Read the model definition and answer for the solid it produces. Units are mm, in the model's axes. Coordinates: 2 decimals unless noted, no trailing zeros. Write each loop counter-clockwise with the first axis right and the second up, starting at its lowest first coordinate (ties: lowest second). Pieces come first, ordered by that corner, then holes.
(1) Straight lines are drawn through the part: line 1 along X through (y, z) = (3.4, 0); line 2 along X through (y, z) = (-3.5, 0.75); line 3 along Z through (x, y) = (-35, 1). For each, find the intervals that lie inside material, in ascending order.
(2) The part is cut by section C-C, the plane y = 1.25. Determine the outline of the cut face in (x, z) (1 decimal).
(3) The part is cut by section A-A, the plane z = 0. Determine the outline of the cut face in (x, y) (1 decimal), and give its area (3 significant figures).
(4) The part is cut by section B-B, the plane x = -8. Determine the outline of the cut face in (y, z) (3 decimals).
(5) Given pin 1 (3 mm diameter, centred on x = -19, z = -3, fed in from +Y); pin 2 (3.5 mm diameter, centred on x = 35.306, z = 0, fed in from +Y) (3 decimals); pin 3 (2 mm diameter, centred on x = 28.5, z = -3, fed in from -Y); pin 4 (1.5 mm diameter, centred on x = -2.5, y = 1, fed in from +Z), each flat-ended and moving along its own axis, determine where each tip first touches the part or whether it passes through.
```python
from build123d import *

# Parameters (mm, degrees)
SKETCH1_R               = 4.445
BOSS_EXTRUDE1_DEPTH     = 38.481
SKETCH2_R               = 1.5875
CUT_EXTRUDE1_DEPTH      = 5.445
CUT_EXTRUDE1_DEPTH_BACK = 5.445


with BuildPart() as part:
    # Sketch1 → Boss-Extrude1 (new body, symmetric)
    with BuildSketch(Plane(origin=(0, 0, 0), x_dir=(0, 0, -1), z_dir=(1, 0, 0))):
        Circle(SKETCH1_R)
    extrude(amount=BOSS_EXTRUDE1_DEPTH, both=True)

    # Sketch2 → Cut-Extrude1 (cut, two sides)
    with BuildSketch(Plane(origin=(0, 0, 0), x_dir=(1, 0, 0), z_dir=(0, 1, 0))) as cut_extrude1_sk:
        with Locations((-35.306, 0)):
            Circle(SKETCH2_R)
        with Locations((35.306, 0)):
            Circle(SKETCH2_R)
    extrude(amount=CUT_EXTRUDE1_DEPTH, mode=Mode.SUBTRACT)
    extrude(cut_extrude1_sk.sketch, amount=-CUT_EXTRUDE1_DEPTH_BACK, mode=Mode.SUBTRACT)


solid = part.part
```
Computed:
1. line 1: x = -38.48 to -36.89, -33.72 to 33.72, 36.89 to 38.48
1. line 2: x = -38.48 to -36.71, -33.91 to 33.91, 36.71 to 38.48
1. line 3: z = -4.33 to -1.56, 1.56 to 4.33
2. outline: (-38.5, -4.3) - (38.5, -4.3) - (38.5, 4.3) - (-38.5, 4.3) - close; hole circle Ø3.2 at (-35.3, 0); hole circle Ø3.2 at (35.3, 0)
3. outline: (-38.5, -4.4) - (-36.9, -4.4) - (-36.9, 4.4) - (-38.5, 4.4) - close; (-33.7, -4.4) - (33.7, -4.4) - (33.7, 4.4) - (-33.7, 4.4) - close; (36.9, -4.4) - (38.5, -4.4) - (38.5, 4.4) - (36.9, 4.4) - close
3. area: 628 mm2
4. outline: circle Ø8.89 at (0, 0)
5. pin 1: stops at y = 4.18
5. pin 2: stops at y = 4.445
5. pin 3: stops at y = -3.97
5. pin 4: stops at z = 4.44
